from build123d import *

# Parameters (mm, degrees)
F0_W     = 118.6410989612
F0_H     = 61.7450922728
F0_W_2   = 91.4861774072
F0_H_2   = 36.5298185498
F1_DEPTH = 50.8
F2_R     = 6.3622008296
F2_R_2   = 5.7887908355
F2_R_3   = 6.6303332555
F3_DEPTH = 48.26
F4_R     = 5.08


with BuildPart() as f1:
    # F0 (on Front) → F1 (new body)
    with BuildSketch(Plane.XZ):
        with Locations((29.2561845854, -7.7603831887)):
            Rectangle(F0_W, F0_H)
        with Locations((30.5492696352, -8.4069287404)):
            Rectangle(F0_W_2, F0_H_2, mode=Mode.SUBTRACT)
    extrude(amount=F1_DEPTH)

    # F2 (on face) → F3 (join)
    with BuildSketch(Plane(origin=(0, 0, 9.8579805344), x_dir=(1, 0, 0), z_dir=(0, 0, -1))):
        with Locations((38.9011949301, 22.1416186541)):
            Circle(F2_R)
        with Locations((60.8952976763, 19.697830081)):
            Circle(F2_R_2)
        with Locations((9.1684339568, 22.548917681)):
            Circle(F2_R_3)
    extrude(amount=F3_DEPTH)

    # F4
    f4_edges = [f1.edges().sort_by_distance(p)[0] for p in [
        (30.54927, -50.8, -26.671838),
    ]]
    fillet(f4_edges, radius=F4_R)


solid = f1.part
Read the model definition and answer for the solid it produces. Units are mm, in the model's axes. A direction names the side the tool comes from. Coordinates: 2 decimals unless noted, no trailing zeros. Loops run counter-clockwise (first coordinate to the right, second up) from the corner with the lowest first, then second, coordinate; pieces in that order, holes last. Notation, with made-up numbers: (33, 8) - (40, 8) arc R23 cw to (40, 16) - close; hole circle Ø11 at (61.25, -7.75). An arc over 180 degrees is marked (long way). Answer in a Markdown table with one row per item.
Q1. The mould has two halves that part along Z. Classify faces 1 (the flat face through (88.577, -25, -8)), 2 (the flat face through (76.292, -25, -11)), 3 (the flat face through (28, -25, 23.112)): pulls with the +Z half, pulls with the -Z half, needs draft (parallel to the pull), parting line crosses it, or undercut.
Here are the results:
| item | result |
|---|---|
| face 1 | needs draft |
| face 2 | undercut |
| face 3 | pulls with the +Z half |
Q2. Find section C-C on z = -14. Write down the section's boundary in (x, y).
Here are the results:
| item | result |
|---|---|
| outline | (-30.06, -50.8) - (-15.19, -50.8) - (-15.19, 0) - (-30.06, 0) - close; circle Ø13.26 at (9.17, -22.55); circle Ø12.72 at (38.9, -22.14); circle Ø11.58 at (60.9, -19.7); (76.29, -50.8) - (88.58, -50.8) - (88.58, 0) - (76.29, 0) - close |
Q3. Find section A-A on y = -40.5. Write down the section's boundary in (x, z), plus the area to 3 significant figures.
Here are the results:
| item | result |
|---|---|
| outline | (-30.06, -38.63) - (88.58, -38.63) - (88.58, 23.11) - (-30.06, 23.11) - close; hole (-15.19, -26.67) - (76.29, -26.67) - (76.29, 9.86) - (-15.19, 9.86) - close |
| area | 3,980 mm^2 |
Q4. Find section B-B on x = 52.5. Write down the section's boundary in (y, z).
Here are the results:
| item | result |
|---|---|
| outline | (-50.8, -38.63) - (0, -38.63) - (0, -26.67) - (-45.72, -26.67) arc R5.08 ccw to (-50.8, -31.75) - close; (-50.8, 9.86) - (0, 9.86) - (0, 23.11) - (-50.8, 23.11) - close |
Q5. Given P1, Ø1.5, axis at x = 13, z = 12, coming from the +Y side, flat-ended and moving along its own axis, determine where the tip first touches the part or whether it passes through.
Here are the results:
| item | result |
|---|---|
| P1 | stops at y = 0 |
Q6. Find section D-D on x = 14. Write down the section's boundary in (y, z).
Here are the results:
| item | result |
|---|---|
| outline | (-50.8, -38.63) - (0, -38.63) - (0, -26.67) - (-18.01, -26.67) - (-18.01, 9.86) - (0, 9.86) - (0, 23.11) - (-50.8, 23.11) - (-50.8, 9.86) - (-27.09, 9.86) - (-27.09, -26.67) - (-45.72, -26.67) arc R5.08 ccw to (-50.8, -31.75) - close |
Q7. For faces 4 (the cylindrical face through (31.19, -49.27, -28.12)), 5 (the flat face through (28, -50.8, 13)), 6 (the cylindrical face through (12.23, -16.67, -8.15)), determine the directions among +Z, -Z, +X, -X, +Y, -Y from which every point of the face is accessible in a straight line to the end or side of a thin tool.
Here are the results:
| item | result |
|---|---|
| face 4 | -Y |
| face 5 | +Z, -Z, +X, -X, -Y |
| face 6 | none |
Q8. Straight lines are drawn through the part: line 1 along X through (y, z) = (-36.5, 5); line 2 along Z through (x, y) = (-9.5, -27); line 3 along X through (y, z) = (-18.5, 6). For each, find the intervals that lie inside material, in ascending order. Write a range as [from, to].
Here are the results:
| item | result |
|---|---|
| line 1 | x = [-30.06, -15.19], [76.29, 88.58] |
| line 2 | z = [-38.63, -26.67], [9.86, 23.11] |
| line 3 | x = [-30.06, -15.19], [3.92, 14.42], [33.68, 44.12], [55.23, 66.56], [76.29, 88.58] |
